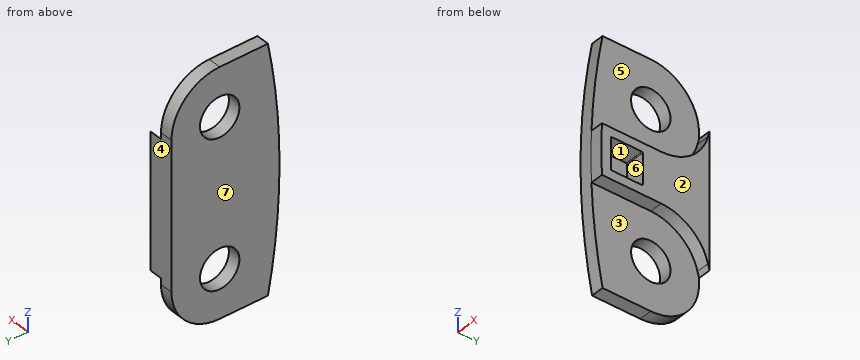
from build123d import *

# Parameters (mm, degrees)
SKETCH004_R  = 2.45
PAD003_DEPTH = 1.6
PAD004_DEPTH = 1.6
POCKET_DEPTH = 2.401


with BuildPart() as part:
    # Sketch004 → Pad003 (new body)
    with BuildSketch(Plane.YZ.offset(-8.7)):
        with BuildLine():
            ThreePointArc((6, 18.2), (4.2426406871, 22.4426406871), (0, 24.2))
            Line((0, 24.2), (-6, 24.2))
            ThreePointArc((-6, 24.2), (-7.4371881489, 9.1), (-6, -6))
            Line((0, -6), (-6, -6))
            ThreePointArc((0, -6), (4.2426406871, -4.2426406871), (6, 0))
            Line((6, 0), (6, 18.2))
        make_face()
        with Locations((0, 18.2)):
            Circle(SKETCH004_R, mode=Mode.SUBTRACT)
        Circle(SKETCH004_R, mode=Mode.SUBTRACT)
    extrude(amount=-PAD003_DEPTH)

    # Sketch005 → Pad004 (join)
    with BuildSketch(Plane.YZ.offset(-8.7)):
        with BuildLine():
            ThreePointArc((0, 12.2), (3.6774423219, 13.4590699257), (5.8114989668, 16.707860677))
            Line((5.8114989668, 16.707860677), (6, 17.4420237293))
            Line((6, 17.4420237293), (6, 0.7579762707))
            Line((6, 0.7579762707), (5.8114989668, 1.492139323))
            ThreePointArc((5.8114989668, 1.492139323), (3.6774423219, 4.7409300743), (0, 6))
            Line((-7.3771358599, 6), (0, 6))
            ThreePointArc((-7.3771358599, 12.2), (-7.4371881489, 9.1), (-7.3771358599, 6))
            Line((-7.3771358599, 12.2), (0, 12.2))
        make_face()
    extrude(amount=PAD004_DEPTH)

    # Sketch065 (on Face1 of Binder015) → Pocket (cut, through all)
    with BuildSketch(Plane(origin=(-9.5, 0, 0), x_dir=(0, -1, 0), z_dir=(-1, 0, 0))):
        with BuildLine():
            Line((6.1771358599, 11.1), (2.4, 11.1))
            ThreePointArc((2.3, 11), (2.3292893219, 11.0707106781), (2.4, 11.1))
            Line((2.3, 11), (2.3, 7.2))
            ThreePointArc((2.4, 7.1), (2.3292893219, 7.1292893219), (2.3, 7.2))
            Line((2.4, 7.1), (6.1771358599, 7.1))
            ThreePointArc((6.2771358599, 7.2), (6.247846538, 7.1292893219), (6.1771358599, 7.1))
            Line((6.2771358599, 7.2), (6.2771358599, 11))
            ThreePointArc((6.1771358599, 11.1), (6.247846538, 11.0707106781), (6.2771358599, 11))
        make_face()
    extrude(amount=-POCKET_DEPTH, mode=Mode.SUBTRACT)


with BuildPart() as part_1:
    # Body005 placement: moved
    add(part.part.moved(Location((0, -72.6064407756, 0))))


solid = part_1.part
Verification items for the finished model (mm, model axes). Face numbers are marked on the shaded views. A direction names the side the tool comes from. Round coordinates to 2 decimals unless told otherwise and drop trailing zeros. Order: outer loops, then holes, each group sorted by start corner. A loop starts at its lowest first (then second) coordinate and runs counter-clockwise, first axis right, second up.
1. Thickness scan on L1, parallel to Z at x = -8.25, y = -78.25; L2, parallel to Z at x = -9.75, y = -70.5; L3, parallel to Z at x = -9.35, y = -77. Record the ranges inside material, lowest first.
Final values:
L1: z = 6 to 7.1, 11.1 to 12.2
L2: z = -5.62 to -1.25, 1.25 to 16.95, 19.45 to 23.82
L3: z = -6 to 7.1, 11.1 to 24.2
2. Access from +Z, -Z, +X, -X, +Y, -Y to the whole of each face (thin tool, end or side, straight path). Record for the marked faces 3, 4, 5, 6 and 7.
Final values:
face 3: -Z, +X, -Y
face 4: +Z, -Z, +X, -X, +Y
face 5: +Z, +X, -Y
face 6: +X
face 7: +Z, -Z, -X, +Y, -Y
3. Section check A-A on x = -7.85. Record the cut outline in (y, z).
Final values:
outline: (-79.98, 6) - (-72.61, 6) arc R6 cw to (-66.79, 1.49) - (-66.61, 0.76) - (-66.61, 17.44) - (-66.79, 16.71) arc R6 cw to (-72.61, 12.2) - (-79.98, 12.2) arc R80.04 ccw to start; hole (-78.88, 7.2) arc R0.1 ccw to (-78.78, 7.1) - (-75.01, 7.1) arc R0.1 ccw to (-74.91, 7.2) - (-74.91, 11) arc R0.1 ccw to (-75.01, 11.1) - (-78.78, 11.1) arc R0.1 ccw to (-78.88, 11) - close
4. Release check for a two-part mould opening along Z. For the marked faces 1 and 2 record: +Z half, -Z half, draft (parallel to the pull), parting line (faces both ways), or undercut.
Final values:
face 1: undercut
face 2: draft
5. Section check C-C on y = -75.5. Record the cut outline in (x, z), then the cut area to 3 significant figures.
Final values:
outline: (-10.3, -6) - (-8.7, -6) - (-8.7, 6) - (-7.1, 6) - (-7.1, 7.1) - (-9.5, 7.1) - (-9.5, 11.1) - (-7.1, 11.1) - (-7.1, 12.2) - (-8.7, 12.2) - (-8.7, 24.2) - (-10.3, 24.2) - close
area: 48.6 mm2
6. Section check D-D on z = 8. Record the cut outline in (x, y).
Final values:
outline: (-10.3, -80.04) - (-7.1, -80.04) - (-7.1, -78.88) - (-9.5, -78.88) - (-9.5, -74.91) - (-7.1, -74.91) - (-7.1, -66.61) - (-10.3, -66.61) - close
7. Section check B-B on z = -0.5. Record the cut outline in (x, y).
Final values:
outline: (-10.3, -79.47) - (-8.7, -79.47) - (-8.7, -75) - (-10.3, -75) - close; (-10.3, -70.21) - (-8.7, -70.21) - (-8.7, -66.63) - (-10.3, -66.63) - close
8. Go/stop test with flat-tipped pins: P1, Ø1, axis at x = -10, z = 3, coming from the -Y side; P2, Ø0.5, axis at x = -8, y = -75, coming from the -Z side; P3, Ø3, axis at y = -77, z = 9, coming from the +X side. Record where each tip stops, or that it passes through.
Final values:
P1: stops at y = -79.85
P2: stops at z = 6
P3: stops at x = -9.5
